from build123d import *

# Parameters (mm, degrees)
F0_R     = 12.5
F1_DEPTH = 53.975
F3_W     = 7
F3_H     = 4.045
F4_DEPTH = 41.276
F6_DEPTH = 3.5


with BuildPart() as f1:
    # F0 (on Right) → F1 (new body)
    with BuildSketch(Plane.YZ):
        Circle(F0_R)
    extrude(amount=F1_DEPTH)

    # F3 (on offset) → F4 (cut, through all)
    with BuildSketch(Plane.YZ.offset(12.7)):
        with Locations((0, 10.4775)):
            Rectangle(F3_W, F3_H)
    extrude(amount=F4_DEPTH, mode=Mode.SUBTRACT)

    # F5 (on Front) → F6 (cut, symmetric)
    with BuildSketch(Plane.XZ):
        Polygon((0, 12.5), (12.7, 8.455), (12.7, 12.5), align=None)
    extrude(amount=F6_DEPTH, both=True, mode=Mode.SUBTRACT)


solid = f1.part
Design review of the part built by this model. Coordinates are the model's own, in mm. A direction names the side the tool comes from. Coordinates: 2 decimals unless noted, no trailing zeros. Order: outer loops, then holes, each group sorted by start corner. A loop starts at its lowest first (then second) coordinate and runs counter-clockwise, first axis right, second up. Notation, with made-up numbers: M 28,42.5 L 71,42.5 A19 ccw 71,58.5 Z; hole C -33,-32.5 d5. An arc over 180 degrees is marked long. Use a Markdown table: item, result.
(1) Add section C-C (y = -7.5). Give the boundary of the cut face in (x, z) (3 decimals).
Worked answers:
| item | result |
|---|---|
| outline | M 0,-10 L 53.975,-10 L 53.975,10 L 0,10 Z |
(2) Add section A-A (z = 10.25). Give the boundary of the cut face in (x, y) (3 decimals).
Worked answers:
| item | result |
|---|---|
| outline | M 0,-7.155 L 53.975,-7.155 L 53.975,-3.5 L 7.064,-3.5 L 7.064,3.5 L 53.975,3.5 L 53.975,7.155 L 0,7.155 Z |
(3) Draft analysis for pull direction Y (two halves, no side actions). For faces 3 (the flat face through (0, 0, 0)), 4 (the flat face through (27, -3.5, 10)), state which applies: released by +Y, released by -Y, zero draft, split by the parting line, or undercut.
Worked answers:
| item | result |
|---|---|
| face 3 | zero draft |
| face 4 | undercut |
(4) Wall thickness on probe 1 along Y at (x, z) = (44, 9.5); probe 2 along Y at (x, z) = (38.5, 8.75); probe 3 along Y at (x, z) = (28.5, -8.75): over which ranges is each line inside the solid? List them lowest first.
Worked answers:
| item | result |
|---|---|
| probe 1 | y = -8.12 to -3.5, 3.5 to 8.12 |
| probe 2 | y = -8.93 to -3.5, 3.5 to 8.93 |
| probe 3 | y = -8.93 to 8.93 |
(5) For faces 1 (the flat face through (53.975, 0, 0)), 2 (the flat face through (27, 3.5, 10)), list the 3-axis set-ups (+Z, -Z, +X, -X, +Y, -Y) from which the entire face can be reached by the end or side of a thin tool; tool diameter is ignored.
Worked answers:
| item | result |
|---|---|
| face 1 | +Z, -Z, +X, +Y, -Y |
| face 2 | +Z, +X |
(6) For P1, Ø1.8, axis at x = 29, z = 10.5, coming from the -Y side; P2, Ø3, axis at x = 24.5, z = 10, coming from the +Y side; P3, Ø7.5, axis at x = 27, y = 1.5, coming from the +Z side, all flat-tipped, find the tip position at first contact; note any pin that passes through.
Worked answers:
| item | result |
|---|---|
| P1 | stops at y = -8.01 |
| P2 | stops at y = 9.17 |
| P3 | stops at z = 12 |
(7) Add section B-B (x = 48). Give the boundary of the cut face in (y, z) (3 decimals), then the cut area to 3 significant figures.
Worked answers:
| item | result |
|---|---|
| outline | M -3.5,8.455 L -3.5,12 A12.5 ccw long 3.5,12 L 3.5,8.455 Z |
| area | 464 mm2 |
